from build123d import *

# Parameters (mm, degrees)
F1_DEPTH = 5
F2_R     = 4.141885
F3_DEPTH = 25
F4_R     = 1


with BuildPart() as f1:
    # F0 (on Top) → F1 (new body)
    with BuildSketch(Plane.XY):
        Polygon((10.952281, 16.452128), (0, 0), (19.723589, 15.361642), (4.361948, 35.085231), align=None)
        Polygon((19.723589, 15.361642), (0, 0), (18.633102, 6.590334), (35.085231, -4.361948), align=None)
        Polygon((39.447178, 30.723283), (19.723589, 15.361642), (35.085231, -4.361948), (28.494897, 14.271155), align=None)
        Polygon((4.361948, 35.085231), (19.723589, 15.361642), (39.447178, 30.723283), (20.814076, 24.132949), align=None)
    extrude(amount=F1_DEPTH)

    # F2 (on face) → F3 (cut)
    with BuildSketch(Plane.XY.offset(5)):
        with Locations((19.723589, 15.361642)):
            Circle(F2_R)
    extrude(amount=-F3_DEPTH, mode=Mode.SUBTRACT)

    # F4
    f4_edges = [f1.edges().sort_by_distance(p)[0] for p in [
        (7.657115, 25.76868, 5),
        (12.588012, 29.60909, 5),
        (5.476141, 8.226064, 5),
        (30.130627, 27.428116, 5),
        (9.316551, 3.295167, 5),
        (33.971038, 22.497219, 5),
        (26.859166, 1.114193, 5),
        (31.790064, 4.954604, 5),
        (15.581704, 15.361642, 5),
        (7.657115, 25.76868, 0),
        (12.588012, 29.60909, 0),
        (5.476141, 8.226064, 0),
        (30.130627, 27.428116, 0),
        (9.316551, 3.295167, 0),
        (33.971038, 22.497219, 0),
        (26.859166, 1.114193, 0),
        (31.790064, 4.954604, 0),
        (15.581704, 15.361642, 0),
        (35.085231, -4.361948, 2.5),
        (28.494897, 14.271155, 2.5),
        (39.447178, 30.723283, 2.5),
        (20.814076, 24.132949, 2.5),
        (4.361948, 35.085231, 2.5),
        (10.952281, 16.452128, 2.5),
        (0, 0, 2.5),
        (18.633102, 6.590334, 2.5),
    ]]
    fillet(f4_edges, radius=F4_R)


solid = f1.part
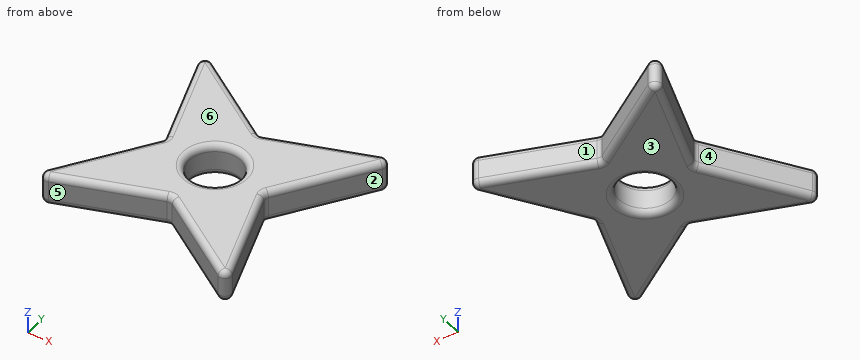
Verification items for the finished model (mm, model axes). Face numbers are marked on the shaded views. A direction names the side the tool comes from. Round coordinates to 2 decimals unless told otherwise and drop trailing zeros. Order: outer loops, then holes, each group sorted by start corner. A loop starts at its lowest first (then second) coordinate and runs counter-clockwise, first axis right, second up.
1. Release check for a two-part mould opening along Y. For the marked faces 1, 2 and 3 record: +Y half, -Y half, draft (parallel to the pull), parting line (faces both ways), or undercut.
Final values:
face 1: +Y half
face 2: undercut
face 3: draft
2. Access from +Z, -Z, +X, -X, +Y, -Y to the whole of each face (thin tool, end or side, straight path). Record for the marked faces 4, 5 and 6.
Final values:
face 4: +Z, -Z, -X
face 5: +Z, -Z, -Y
face 6: +Z, +X, -X, +Y, -Y
3. Section check A-A on z = 3.45. Record the cut outline in (x, y), then the cut area to 3 significant figures.
Final values:
outline: (1.66, 2.5) arc R1 ccw to (2.83, 1) - (18.16, 6.42) arc R1 cw to (19.05, 6.31) - (32.59, -2.7) arc R1 ccw to (34.08, -1.53) - (28.66, 13.8) arc R1 cw to (28.77, 14.69) - (37.78, 28.23) arc R1 ccw to (36.62, 29.72) - (21.29, 24.3) arc R1 cw to (20.4, 24.41) - (6.86, 33.42) arc R1 ccw to (5.36, 32.26) - (10.79, 16.92) arc R1 cw to (10.68, 16.04) - close; hole circle Ø8.28 at (19.72, 15.36)
area: 564 mm2
4. Go/stop test with flat-tipped pins: P1, Ø1, axis at y = 26, z = 1, coming from the +X side; P2, Ø3, axis at y = 13, z = 1, coming from the +X side (3 decimals). Record where each tip stops, or that it passes through.
Final values:
P1: stops at x = 36.64
P2: stops at x = 29.475
5. Thickness scan on L1, parallel to Y at x = 17, z = 0.35; L2, parallel to Y at x = 19, z = 0.85; L3, parallel to X at y = 12, z = 0.3. Record the ranges inside material, lowest first.
Final values:
L1: y = 6.27 to 11.93, 18.79 to 26.38
L2: y = 6.36 to 11.27, 19.45 to 25.33
L3: x = 8.33 to 16.84, 22.61 to 28.99
